```python
from build123d import *

# Parameters (mm, degrees)
SKETCH_1_R          = 1.5
EXTRUDE_1_DEPTH     = 3
SKETCH_4_R          = 1.5
CUT_EXTRUDE_1_DEPTH = 3
SKETCH_6_W          = 6
SKETCH_6_H          = 20
EXTRUDE_2_DEPTH     = 3
FILLET_1_R          = 2


with BuildPart() as part:
    # 草图1 → 凸台-拉伸1 (new body)
    with BuildSketch(Plane.XY):
        Polygon((-14, -10), (-0.55, -17), (-0.55, -52), (5.45, -52), (14, -10), (14, 10), (-14, 10), align=None)
        with Locations((5, 7.5)):
            Circle(SKETCH_1_R, mode=Mode.SUBTRACT)
        with Locations((5, -7.5)):
            Circle(SKETCH_1_R, mode=Mode.SUBTRACT)
        with Locations((-5, -7.5)):
            Circle(SKETCH_1_R, mode=Mode.SUBTRACT)
        with Locations((-5, 7.5)):
            Circle(SKETCH_1_R, mode=Mode.SUBTRACT)
    extrude(amount=EXTRUDE_1_DEPTH)

    # 草图4 → 切除-拉伸1 (cut)
    with BuildSketch(Plane.XY.offset(3)):
        with Locations((2.45, -37)):
            Circle(SKETCH_4_R)
        with Locations((2.45, -17)):
            Circle(SKETCH_4_R)
    extrude(amount=-CUT_EXTRUDE_1_DEPTH, mode=Mode.SUBTRACT)

    # 草图6 → 凸台-拉伸2 (add)
    with BuildSketch(Plane.XY.offset(3)):
        with Locations((17, 0)):
            Rectangle(SKETCH_6_W, SKETCH_6_H)
    extrude(amount=-EXTRUDE_2_DEPTH)

    # 圆角1
    fillet_1_edges = [part.edges().sort_by_distance(p)[0] for p in [
        (-0.55, -52, 1.5),
        (-0.55, -17, 1.5),
        (-14, -10, 1.5),
        (-14, 10, 1.5),
        (14, -10, 1.5),
        (5.45, -52, 1.5),
        (20, 10, 1.5),
        (20, -10, 1.5),
    ]]
    fillet(fillet_1_edges, radius=FILLET_1_R)


solid = part.part
```
Read the model definition and answer for the solid it produces. Units are mm, in the model's axes. A direction names the side the tool comes from. Give positions to 0.01 mm unless a question says otherwise; leave off trailing zeros. Write each loop counter-clockwise with the first axis right and the second up, starting at its lowest first coordinate (ties: lowest second). Pieces come first, ordered by that corner, then holes. Notation, with made-up numbers: (-33, 45.25) -> (-6, 45.25) arc R25 cw to (-6, 80.25) -> close; hole circle Ø5 at (59, 81). An arc over 180 degrees is marked (long way). Answer as a JSON object with one key per item and string values.
1) A tool of negligible diameter and unlimited length cuts with its end or side. For faces 4 (the flat face through (3, -7, 3)), 5 (the flat face through (-0.55, -34, 1)), from which of +Z, -Z, +X, -X, +Y, -Y can it reach the whole face along a straight path? Write none if from no direction.
Findings below:
{"face 4": "+Z, +X, -X, +Y, -Y", "face 5": "+Z, -Z, -X, -Y"}
2) Section D-D on x = -5 is taken. Write down the section's boundary in (y, z), then the cut area to 3 significant figures.
Findings below:
{"outline": "(-14.68, 0) -> (-9, 0) -> (-9, 3) -> (-14.68, 3) -> close; (-6, 0) -> (6, 0) -> (6, 3) -> (-6, 3) -> close; (9, 0) -> (10, 0) -> (10, 3) -> (9, 3) -> close", "area": "56.1 mm^2"}
3) Flat-ended cylindrical pins translate along their axes: pin 1 Ø1.5 at (y, z) = (-37.5, 1) entering from -X; pin 2 Ø1.2 at (x, z) = (17, 1.5) entering from -Y; pin 3 Ø1.5 at (y, z) = (-45.5, 1.5) entering from -X; pin 4 Ø5 at (x, y) = (5, -7.5) entering from -Z. Find the tip coordinate at first contact, or state that the pin passes through.
Findings below:
{"pin 1": "stops at x = -0.55", "pin 2": "stops at y = -10", "pin 3": "stops at x = -0.55", "pin 4": "stops at z = 0"}
4) For a pull along X with two mould halves and no side action, classify faces 1 (the cylindrical face through (2.125, -38.464, 1.521)), 2 (the cylindrical face through (19.4, 9.43, 1.48)), 3 (the cylindrical face through (-13.7, -9.84, 1.52)) as pulls with the +X half, pulls with the -X half, needs draft (parallel to the pull), parting line crosses it, or undercut.
Findings below:
{"face 1": "undercut", "face 2": "pulls with the +X half", "face 3": "pulls with the -X half"}
5) Straight lines are drawn through the part: probe 1 along Y at (x, z) = (2.45, 0.7); probe 2 along Y at (x, z) = (5, 2.15); probe 3 along Y at (x, z) = (17, 1.1). For each, find the intervals that lie inside material, in ascending order. Write a range as from..to.
Findings below:
{"probe 1": "y = -52..-38.5, -35.5..-18.5, -15.5..10", "probe 2": "y = -51.61..-9, -6..6, 9..10", "probe 3": "y = -10..10"}
6) Section B-B on z = 2.25 is taken. Write down the section's boundary in (x, y), then the cut area to 3 significant figures.
Findings below:
{"outline": "(-14, -8.79) arc R2 ccw to (-12.92, -10.56) -> (-1.63, -16.44) arc R2 cw to (-0.55, -18.21) -> (-0.55, -50) arc R2 ccw to (1.45, -52) -> (3.82, -52) arc R2 ccw to (5.78, -50.4) -> (13.67, -11.6) arc R2 cw to (15.63, -10) -> (18, -10) arc R2 ccw to (20, -8) -> (20, 8) arc R2 ccw to (18, 10) -> (-12, 10) arc R2 ccw to (-14, 8) -> close; hole circle Ø3 at (-5, -7.5); hole circle Ø3 at (-5, 7.5); hole circle Ø3 at (2.45, -37); hole circle Ø3 at (2.45, -17); hole circle Ø3 at (5, -7.5); hole circle Ø3 at (5, 7.5)", "area": "1,110 mm^2"}
7) Section A-A on x = 2.45 is taken. Write down the section's boundary in (y, z).
Findings below:
{"outline": "(-52, 0) -> (-38.5, 0) -> (-38.5, 3) -> (-52, 3) -> close; (-35.5, 0) -> (-18.5, 0) -> (-18.5, 3) -> (-35.5, 3) -> close; (-15.5, 0) -> (10, 0) -> (10, 3) -> (-15.5, 3) -> close"}
8) Section C-C on y = -37 is taken. Write down the section's boundary in (x, z).
Findings below:
{"outline": "(-0.55, 0) -> (0.95, 0) -> (0.95, 3) -> (-0.55, 3) -> close; (3.95, 0) -> (8.5, 0) -> (8.5, 3) -> (3.95, 3) -> close"}
